```python
from build123d import *

# Parameters (mm, degrees)
SKETCH_1_W          = 50
SKETCH_1_H          = 45
EXTRUDE_1_DEPTH     = 4
SKETCH_2_R          = 2.1
CUT_EXTRUDE_1_DEPTH = 5
SKETCH_5_R          = 2.1
CUT_EXTRUDE_4_DEPTH = 5


with BuildPart() as part:
    # 草图1 → 凸台-拉伸1 (new body)
    with BuildSketch(Plane(origin=(0, 0, 0), x_dir=(1, 0, 0), z_dir=(0, 1, 0))):
        Rectangle(SKETCH_1_W, SKETCH_1_H)
    extrude(amount=EXTRUDE_1_DEPTH)

    # 草图2 → 切除-拉伸1 (cut, through all)
    with BuildSketch(Plane(origin=(0, 4, 0), x_dir=(1, 0, 0), z_dir=(0, 1, 0))):
        with Locations((0, -11)):
            Circle(SKETCH_2_R)
        with Locations((8, -11)):
            Circle(SKETCH_2_R)
        with Locations((-8, -11)):
            Circle(SKETCH_2_R)
    extrude(amount=-CUT_EXTRUDE_1_DEPTH, mode=Mode.SUBTRACT)

    # 草图5 → 切除-拉伸4 (cut, through all)
    with BuildSketch(Plane(origin=(0, 0, 0), x_dir=(-1, 0, 0), z_dir=(0, -1, 0))):
        with Locations((20, -17.5)):
            Circle(SKETCH_5_R)
        with Locations((20, 17.5)):
            Circle(SKETCH_5_R)
        with Locations((-20, 17.5)):
            Circle(SKETCH_5_R)
        with Locations((-20, -17.5)):
            Circle(SKETCH_5_R)
    extrude(amount=-CUT_EXTRUDE_4_DEPTH, mode=Mode.SUBTRACT)


solid = part.part
```
Geometry check sheet. Reference: the model listing, model coordinates, mm. Round coordinates to 2 decimals unless told otherwise and drop trailing zeros. Order: outer loops, then holes, each group sorted by start corner. A loop starts at its lowest first (then second) coordinate and runs counter-clockwise, first axis right, second up. Notation, with made-up numbers: (49, 89.25) - (88, 89.25) arc R19 ccw to (88, 102.25) - close; hole circle Ø4 at (85, 71). An arc over 180 degrees is marked (long way). Use a Markdown table: item, result. Add a question column.
(1) Material ranges on line 1 along X through (y, z) = (2.95, 11); line 2 along X through (y, z) = (1.05, 17.5); line 3 along Z through (x, y) = (-20, 1.8), recorded low to high. Write a range as [from, to].
(2) Sectioned sample at D-D, the plane z = 17.5. Enter the section's corners in (x, y).
(3) Sectioned sample at B-B, the plane x = 20. Enter the section's corners in (y, z).
(4) Sectioned sample at A-A, the plane x = 0. Enter the section's corners in (y, z), and give its area (3 significant figures).
(5) Depth check by flat-ended pin: pin 1 (4 mm diameter, centred on x = -20, z = 17.5, fed in from +Y). Enter the tip coordinate at first touch or a pass-through.
(6) Sectioned sample at C-C, the plane y = 0.7. Enter the section's corners in (x, z), and give its area (3 significant figures).
(7) Release check for a two-part mould opening along X. For faces 1 (the flat face through (0, 4, 0)), 2 (the flat face through (25, 2, 0)), 3 (the cylindrical face through (-22.003, 1.972, 16.869)) record: pulls with the +X half, pulls with the -X half, needs draft (parallel to the pull), parting line crosses it, or undercut.
Answers below:
| question | item | result |
|---|---|---|
| 1 | line 1 | [-25, -10.1], [-5.9, -2.1], [2.1, 5.9], [10.1, 25] |
| 1 | line 2 | [-25, -22.1], [-17.9, 17.9], [22.1, 25] |
| 1 | line 3 | [-22.5, -19.6], [-15.4, 15.4], [19.6, 22.5] |
| 2 | outline | (-25, 0) - (-22.1, 0) - (-22.1, 4) - (-25, 4) - close; (-17.9, 0) - (17.9, 0) - (17.9, 4) - (-17.9, 4) - close; (22.1, 0) - (25, 0) - (25, 4) - (22.1, 4) - close |
| 3 | outline | (0, -22.5) - (4, -22.5) - (4, -19.6) - (0, -19.6) - close; (0, -15.4) - (4, -15.4) - (4, 15.4) - (0, 15.4) - close; (0, 19.6) - (4, 19.6) - (4, 22.5) - (0, 22.5) - close |
| 4 | outline | (0, -22.5) - (4, -22.5) - (4, 8.9) - (0, 8.9) - close; (0, 13.1) - (4, 13.1) - (4, 22.5) - (0, 22.5) - close |
| 4 | area | 163 mm² |
| 5 | pin 1 | through |
| 6 | outline | (-25, -22.5) - (25, -22.5) - (25, 22.5) - (-25, 22.5) - close; hole circle Ø4.2 at (-20, -17.5); hole circle Ø4.2 at (-20, 17.5); hole circle Ø4.2 at (-8, 11); hole circle Ø4.2 at (0, 11); hole circle Ø4.2 at (8, 11); hole circle Ø4.2 at (20, -17.5); hole circle Ø4.2 at (20, 17.5) |
| 6 | area | 2,150 mm² |
| 7 | face 1 | needs draft |
| 7 | face 2 | pulls with the +X half |
| 7 | face 3 | undercut |
